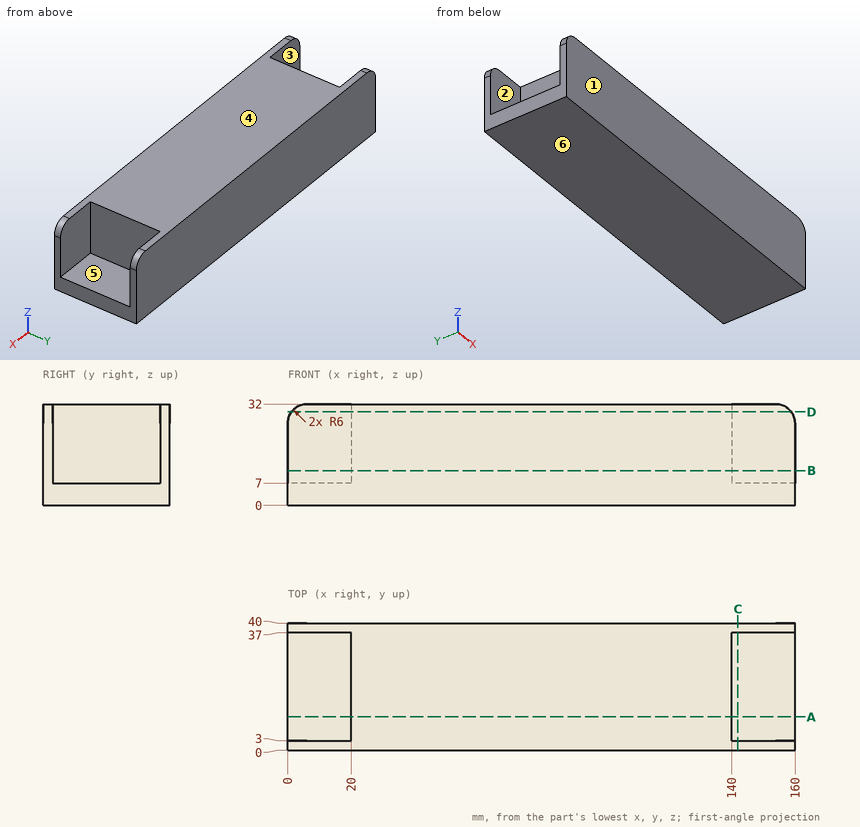
Answer from the drawing. Dimensions are ordinates in mm from the lowest x, y and z of the part. A direction names the side the tool comes from. Coordinates: 2 decimals unless noted, no trailing zeros. Order: outer loops, then holes, each group sorted by start corner. A loop starts at its lowest first (then second) coordinate and runs counter-clockwise, first axis right, second up. Notation, with made-up numbers: (20, 73.25) - (72, 73.25) arc R28 ccw to (72, 92.25) - close; hole circle Ø5 at (35, 81). An arc over 180 degrees is marked (long way). Put each result on its own line as item: value. Start each with the question number.
1) Find section B-B (z = 11). Give the vertices of the cut face in (x, y), plus the area to 3 significant figures.
2) For a pull along Y with two mould halves and no side action, classify the marked faces 1, 2, 3 and 4 as released by +Y, released by -Y, zero draft, split by the parting line, or undercut.
3) Find the intervals of material crossed by line 1 (Y direction, x = 141, z = 13); line 2 (X direction, y = 28, z = 27.5); line 3 (Z direction, x = 16, y = 23), in increasing order. Write a range as from..to.
4) Flat-ended cylindrical pins translate along their axes: pin 1 (1 mm diameter, centred on y = 13, z = 25, fed in from -X); pin 2 (10 mm diameter, centred on x = 148.5, y = 25.5, fed in from +Z); pin 3 (12.5 mm diameter, centred on y = 13, z = 23, fed in from +X). Find the tip coordinate at first contact, or state that the pin passes through.
5) For the marked faces 5 and 6, determine the directions among +Z, -Z, +X, -X, +Y, -Y from which every point of the face is accessible in a straight line to the end or side of a thin tool.
6) Find section A-A (y = 10.5). Give the vertices of the cut face in (x, z), plus the area to 3 significant figures.
7) Find section D-D (z = 29.5). Give the vertices of the cut face in (x, y), plus the area to 3 significant figures.
8) Find section C-C (x = 142). Give the vertices of the cut face in (y, z), plus the area to 3 significant figures.
Results list:
1. outline: (0, 0) - (160, 0) - (160, 3) - (140, 3) - (140, 37) - (160, 37) - (160, 40) - (0, 40) - (0, 37) - (20, 37) - (20, 3) - (0, 3) - close
1. area: 5,040 mm^2
2. face 1: released by -Y
2. face 2: undercut
2. face 3: undercut
2. face 4: zero draft
3. line 1: y = 0..3, 37..40
3. line 2: x = 20..140
3. line 3: z = 0..7
4. pin 1: stops at x = 20
4. pin 2: stops at z = 7
4. pin 3: stops at x = 140
5. face 5: +Z, +X
5. face 6: -Z, +X, -X, +Y, -Y
6. outline: (0, 0) - (160, 0) - (160, 7) - (140, 7) - (140, 32) - (20, 32) - (20, 7) - (0, 7) - close
6. area: 4,120 mm^2
7. outline: (1.13, 0) - (158.87, 0) - (158.87, 3) - (140, 3) - (140, 37) - (158.87, 37) - (158.87, 40) - (1.13, 40) - (1.13, 37) - (20, 37) - (20, 3) - (1.13, 3) - close
7. area: 5,030 mm^2
8. outline: (0, 0) - (40, 0) - (40, 32) - (37, 32) - (37, 7) - (3, 7) - (3, 32) - (0, 32) - close
8. area: 430 mm^2
